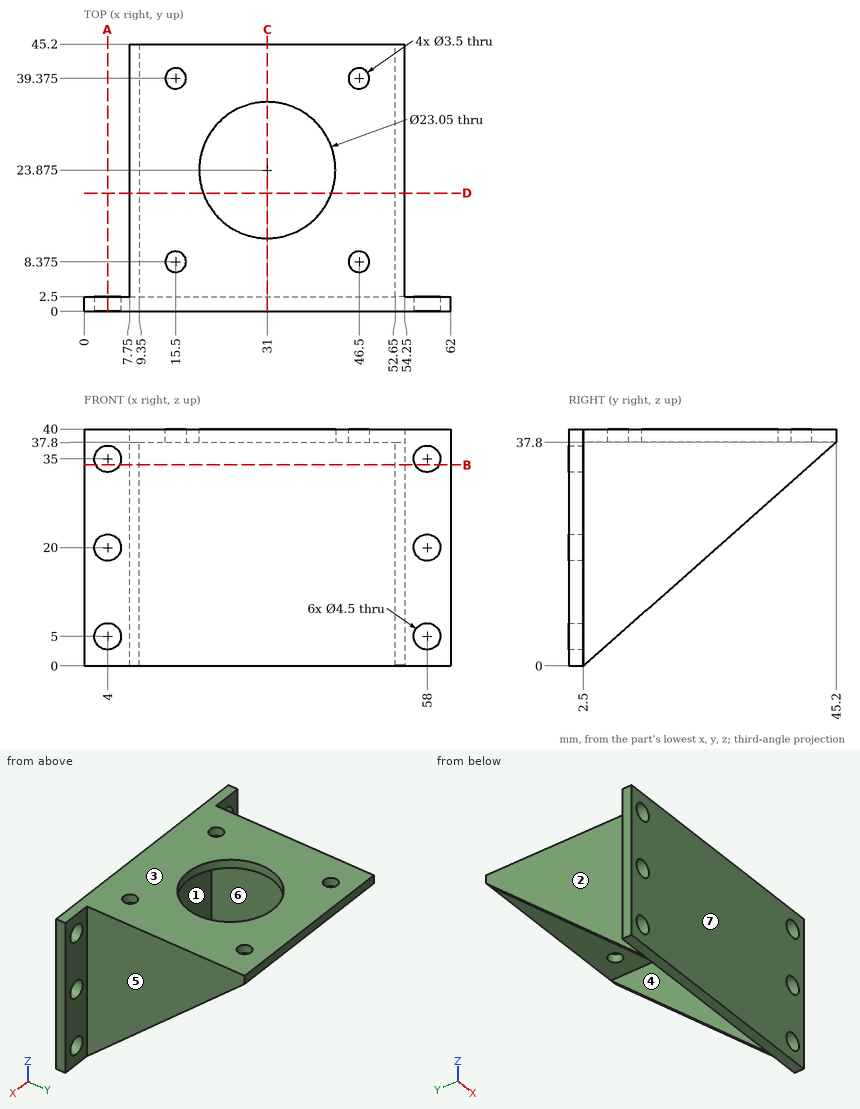
Input: dimensioned drawing with shaded views. Units: mm. Origin: part minimum x, y, z. A direction names the side the tool comes from. Coordinates: 2 decimals unless noted, no trailing zeros. Write each loop counter-clockwise with the first axis right and the second up, starting at its lowest first coordinate (ties: lowest second). Pieces come first, ordered by that corner, then holes. Notation, with made-up numbers: M 80,3 L 115,3 A6 cw 115,11 Z; hole C 33.25,9 d3. An arc over 180 degrees is marked long. Answer as a JSON object with one key per item and string values. Group by question number.
(1) Section B-B on z = 34. Output: boundary loops of the cut face in (x, y), plus the area to 3 significant figures.
(2) Section C-C on x = 31. Output: boundary loops of the cut face in (y, z).
(3) Section D-D on y = 20. Output: boundary loops of the cut face in (x, z).
(4) Mould query, pull axis X, two halves, no side actions, for the marked faces 1, 2, 3 and 4. Classes: pulls with the +X half, pulls with the -X half, needs draft (parallel to the pull), parting line crosses it, or undercut.
(5) Section A-A on x = 4. Output: boundary loops of the cut face in (y, z).
(6) Contact query for flat-ended pins moving along their axis: P1, Ø4, axis at x = 58, z = 35, coming from the +Y side; P2, Ø20, axis at y = 21, z = 27, coming from the -X side; P3, Ø2.5, axis at x = 58, z = 29.5, coming from the +Y side; P4, Ø10, axis at x = 43, y = 38, coming from the -Z side. Output: stop coordinate, or through.
(7) Ray query, line 1 along X through (y, z) = (12, 30); line 2 along X through (y, z) = (1.25, 35); line 3 along Y through (x, z) = (15, 38). Return the intervals inside material, ascending. Write a range as [from, to].
(8) Set-up query: the marked faces 5, 6 and 7. Return all of +Z, -Z, +X, -X, +Y, -Y with unobstructed straight access to the full face (end or side cutting, diameter ignored); none if empty.
Result set:
{
 "1": {"outline": "M 0,0 L 1.98,0 L 1.98,2.5 L 0,2.5 Z; M 6.02,0 L 55.98,0 L 55.98,2.5 L 54.25,2.5 L 54.25,40.91 L 52.65,40.91 L 52.65,2.5 L 9.35,2.5 L 9.35,40.91 L 7.75,40.91 L 7.75,2.5 L 6.02,2.5 Z; M 60.02,0 L 62,0 L 62,2.5 L 60.02,2.5 Z", "area": "258 mm2"},
 "2": {"outline": "M 0,0 L 2.5,0 L 2.5,37.8 L 12.35,37.8 L 12.35,40 L 0,40 Z; M 35.4,37.8 L 45.2,37.8 L 45.2,40 L 35.4,40 Z"},
 "3": {"outline": "M 7.75,15.49 L 9.35,15.49 L 9.35,37.8 L 20.15,37.8 L 20.15,40 L 7.75,40 Z; M 41.85,37.8 L 52.65,37.8 L 52.65,15.49 L 54.25,15.49 L 54.25,40 L 41.85,40 Z"},
 "4": {"face 1": "undercut", "face 2": "pulls with the -X half", "face 3": "needs draft", "face 4": "undercut"},
 "5": {"outline": "M 0,0 L 2.5,0 L 2.5,2.75 L 0,2.75 Z; M 0,7.25 L 2.5,7.25 L 2.5,17.75 L 0,17.75 Z; M 0,22.25 L 2.5,22.25 L 2.5,32.75 L 0,32.75 Z; M 0,37.25 L 2.5,37.25 L 2.5,40 L 0,40 Z"},
 "6": {"P1": "passes through", "P2": "stops at x = 7.75", "P3": "stops at y = 2.5", "P4": "stops at z = 37.8"},
 "7": {"line 1": "x = [7.75, 9.35], [52.65, 54.25]", "line 2": "x = [0, 1.75], [6.25, 55.75], [60.25, 62]", "line 3": "y = [0, 6.7], [10.05, 37.7], [41.05, 45.2]"},
 "8": {"face 5": "+Z, -Z, +X, +Y", "face 6": "-Z, +Y", "face 7": "+Z, -Z, +X, -X, -Y"}
}
